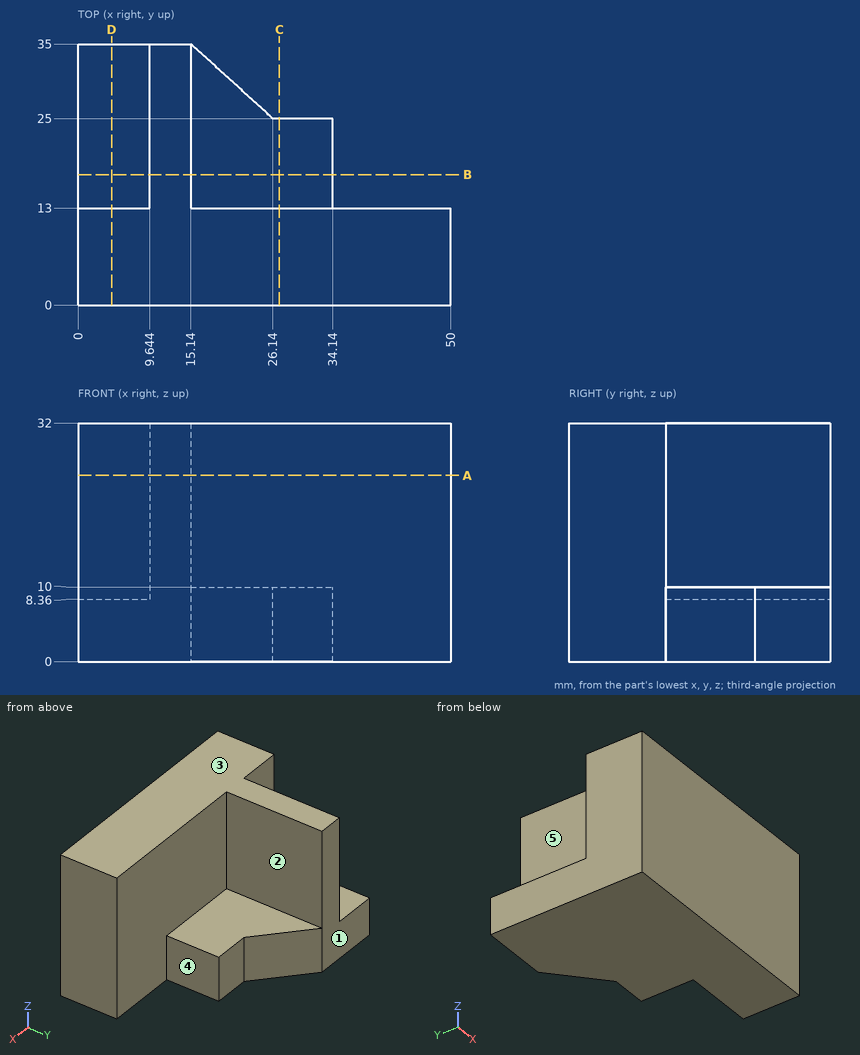
The drawing under review shows one solid part. Ordinate dimensions are in mm from its lowest x, y, z. A direction names the side the tool comes from. Round coordinates to 2 decimals unless told otherwise and drop trailing zeros. Write each loop counter-clockwise with the first axis right and the second up, starting at its lowest first coordinate (ties: lowest second). Pieces come first, ordered by that corner, then holes. Notation, with made-up numbers: (3.5, -9) - (46.5, -9) arc R14 cw to (46.5, 6) - close; hole circle Ø6 at (-39, -19). An arc over 180 degrees is marked (long way). Write each question's results on one line, items separated by ' | '.
Item 1: Take a section at B-B on y = 17.5. State the section outline as (x, z) points.
Calculated:
outline: (0, 0) - (34.14, 0) - (34.14, 10) - (15.14, 10) - (15.14, 32) - (9.64, 32) - (9.64, 8.36) - (0, 8.36) - close
Item 2: To check wall thickness, follow line 1 along X through (y, z) = (30.5, 14); line 2 along Y through (x, z) = (39, 17.5); line 3 along X through (y, z) = (22, 5). State the ranges of each line that lie inside material, in increasing order. Write a range as from..to.
Calculated:
line 1: x = 9.64..15.14 | line 2: y = 0..13 | line 3: x = 0..34.14
Item 3: For the marked faces 1, 2, 3, 4 and 5, list the 3-axis set-ups (+Z, -Z, +X, -X, +Y, -Y) from which the entire face can be reached by the end or side of a thin tool; tool diameter is ignored.
Calculated:
face 1: +Z, -Z, +X, -X, +Y | face 2: +Z, +X, +Y | face 3: +Z, +X, -X, +Y, -Y | face 4: +Z, -Z, +X, +Y | face 5: +Z, -X, +Y
Item 4: Take a section at C-C on x = 27. State the section outline as (y, z) points.
Calculated:
outline: (0, 0) - (25, 0) - (25, 10) - (13, 10) - (13, 32) - (0, 32) - close
Item 5: Take a section at D-D on x = 4.5. State the section outline as (y, z) points, then the cut area to 3 significant figures.
Calculated:
outline: (0, 0) - (35, 0) - (35, 8.36) - (13, 8.36) - (13, 32) - (0, 32) - close | area: 600 mm^2
Item 6: Take a section at A-A on z = 25. State the section outline as (x, y) points.
Calculated:
outline: (0, 0) - (50, 0) - (50, 13) - (15.14, 13) - (15.14, 35) - (9.64, 35) - (9.64, 13) - (0, 13) - close
Item 7: For pin 1 (6.5 mm diameter, centred on y = 20, z = 25.5, fed in from -X); pin 2 (4 mm diameter, centred on x = 29.5, z = 3.5, fed in from +Y); pin 3 (8 mm diameter, centred on x = 29.5, z = 14.5, fed in from +Y), all flat-tipped, find the tip position at first contact; note any pin that passes through.
Calculated:
pin 1: stops at x = 9.64 | pin 2: stops at y = 25 | pin 3: stops at y = 13
